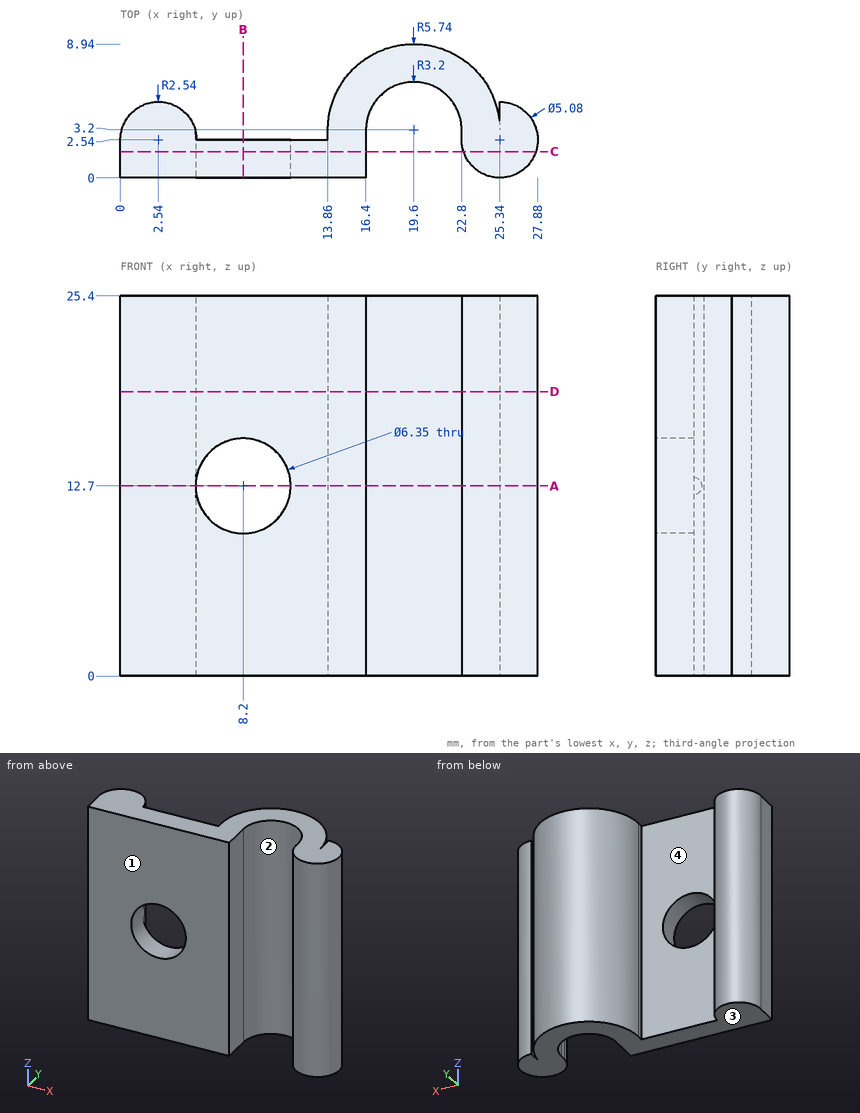
Here's the drawing with two shaded views (mm, measured from the low corner). I have some questions. A direction names the side the tool comes from. Give positions to 0.01 mm unless a question says otherwise; leave off trailing zeros. Write each loop counter-clockwise with the first axis right and the second up, starting at its lowest first coordinate (ties: lowest second). Pieces come first, ordered by that corner, then holes. Notation, with made-up numbers: (58, 69) - (113, 69) arc R14 cw to (113, 80) - close; hole circle Ø5 at (34, 30.25). An arc over 180 degrees is marked (long way). One line per item, written item: value. Start each with the question number.
Item 1: Please list where these lines run through material, in increasing order: line 1 (X direction, y = 1, z = 10.75); line 2 (Z direction, x = 8.2, y = 0.75) (3 decimals); line 3 (X direction, y = 0.75, z = 12). Write a range as from..to.
Item 2: Imagine slicing it at C-C, the plane y = 1.75. List the corners of the cut face in (x, z) for me (3 decimals).
Item 3: Which directions (+Z, -Z, +X, -X, +Y, -Y) give clear straight access to the entire face, cutting with the end or side of a thin tool? Please do the marked faces 3 and 4.
Item 4: If we mould it in two halves opening along X, with no side actions, what happens to the marked faces 1 and 2? For each: +X half, -X half, draft (parallel to the pull), parting line (faces both ways), or undercut.
Item 5: Imagine slicing it at D-D, the plane z = 19. List the corners of the cut face in (x, y) for me.
Item 6: Imagine slicing it at B-B, the plane x = 8.2. List the corners of the cut face in (y, z) for me (3 decimals).
Item 7: I'm going to push flat-ended pins straight in: pin 1 (1.6 mm diameter, centred on y = 2, z = 11, fed in from +X); pin 2 (9.5 mm diameter, centred on x = 8.5, z = 16, fed in from +Y); pin 3 (5 mm diameter, centred on x = 13.5, z = 13, fed in from +Y); pin 4 (1.5 mm diameter, centred on y = 4.5, z = 13, fed in from -X). Where does each tip first touch, or does it pass through?
Item 8: Imagine slicing it at A-A, the plane z = 12.7. List the corners of the cut face in (x, y) for me (3 decimals).
Geometry says:
1. line 1: 0..5.69, 10.71..16.4, 23.32..27.36
1. line 2: 0..9.525, 15.875..25.4
1. line 3: 0..5.1, 11.3..16.4, 23.54..27.14
2. outline: (0, 0) - (16.4, 0) - (16.4, 25.4) - (0, 25.4) - close; (22.926, 0) - (27.754, 0) - (27.754, 25.4) - (22.926, 25.4) - close; hole circle Ø6.35 at (8.2, 12.7)
3. face 3: -Z, +X, -X, +Y, -Y
3. face 4: +Z, -Z, +Y
4. face 1: draft
4. face 2: undercut
5. outline: (0, 0) - (16.4, 0) - (16.4, 3.2) arc R3.2 cw to (22.8, 3.2) - (22.8, 2.54) arc R2.54 ccw (long way) to (25.34, 5.08) - (25.34, 3.2) arc R5.74 ccw to (13.86, 3.2) - (13.86, 2.54) - (5.08, 2.54) arc R2.54 ccw to (0, 2.54) - close
6. outline: (0, 0) - (2.54, 0) - (2.54, 9.525) - (0, 9.525) - close; (0, 15.875) - (2.54, 15.875) - (2.54, 25.4) - (0, 25.4) - close
7. pin 1: x = 27.88
7. pin 2: y = 4.77
7. pin 3: y = 7.67
7. pin 4: x = 0.31
8. outline: (0, 0) - (5.025, 0) - (5.025, 3.066) arc R2.54 ccw to (0, 2.54) - close; (11.375, 0) - (16.4, 0) - (16.4, 3.2) arc R3.2 cw to (22.8, 3.2) - (22.8, 2.54) arc R2.54 ccw (long way) to (25.34, 5.08) - (25.34, 3.2) arc R5.74 ccw to (13.86, 3.2) - (13.86, 2.54) - (11.375, 2.54) - close
